Check sheet for the modelled part. Datum: model origin and axes. Units: mm. A direction names the side the tool comes from. Give positions to 0.01 mm unless a question says otherwise; leave off trailing zeros. Order: outer loops, then holes, each group sorted by start corner. A loop starts at its lowest first (then second) coordinate and runs counter-clockwise, first axis right, second up.
Autodesk Fusion 360 part; units mm, degrees
sketch "Esboço1" plane through (0, 0, 0) normal (0, 0, 1) x (1, 0, 0)
  circle A0 centre (0, 0) radius 3
  dimension "d1" = 6
extrude "Extrusão1" add sketch "Esboço1" along normal blind 40
sketch "Esboço2" plane through (0, 0, 40) normal (0, 0, 1) x (1, 0, 0)
  circle A0 centre (0, 0) radius 3
  circle A1 centre (0, 0) radius 2
  dimension "d4" = 4
extrude "Extrusão2" cut sketch "Esboço2" against normal blind 4 contours A1
extrude "Extrusão3" cut 1 faces at (-1.1591, 0.5829, 0) along direction (0, 0, 1) blind 10
extrude "Extrusão4" cut 1 faces at (0.637, 0.1965, 36) along direction (0, 0, -1) blind 1
chamfer "Chanfro1" distance 0.4 angle 45 1 edges at (-1.8647, 0.7232, 40)
sketch "Esboço3" plane through (0, 0, 10) normal (0, 0, -1) x (-1, 0, 0)
  circle A0 centre (0, 0) radius 3
  circle A1 centre (0, 0) radius 1.4
  dimension "d12" = 2.8
extrude "Extrusão5" cut sketch "Esboço3" against normal blind 10 contours A1
sketch "Esboço4" plane through (0, 0, 10) normal (0, 0, -1) x (-1, 0, 0)
  circle A0 centre (0, 0) radius 1.4
  circle A1 centre (0, 0) radius 3
  circle A2 centre (0, 0) radius 3
  circle A3 centre (0, 0) radius 2.75
  dimension "d15" = 5.5
extrude "Extrusão6" cut sketch "Esboço4" against normal blind 34 contours A1 A2
extrude "Extrusão7" cut 1 faces at (0.637, 0.1965, 35) along direction (0, 0, -1) blind 1
1) Material ranges on L1, parallel to Y at x = 0, z = 36.4; L2, parallel to Y at x = 0, z = 13.75; L3, parallel to Z at x = -1.5, y = 0.45, recorded low to high.
Recorded:
L1: y = -2.75 to -2, 2 to 2.75
L2: y = -2.75 to -1.4, 1.4 to 2.75
L3: z = 10 to 34
2) Section check C-C, the plane z = 33.25. Record the cut outline in (x, y).
Recorded:
outline: circle Ø5.5 at (0, 0)
3) Section check A-A, the plane x = 0. Record the cut outline in (y, z).
Recorded:
outline: (-2.75, 10) - (-1.4, 10) - (-1.4, 20) - (1.4, 20) - (1.4, 10) - (2.75, 10) - (2.75, 40) - (2.4, 40) - (2, 39.6) - (2, 34) - (-2, 34) - (-2, 39.6) - (-2.4, 40) - (-2.75, 40) - close
4) Section check D-D, the plane z = 12.5. Record the cut outline in (x, y), then the cut area to 3 significant figures.
Recorded:
outline: circle Ø5.5 at (0, 0); hole circle Ø2.8 at (0, 0)
area: 17.6 mm2
5) Draft check along X on faces 3 (the face through (0, 0, 20)), 4 (the face through (0.596, -2.685, 24.79)), 5 (the face through (1.2, -1.2, 10)). Enter one of: +X half, -X half, draft (parallel to the pull), parting line (faces both ways), or undercut.
Recorded:
face 3: undercut
face 4: parting line
face 5: draft
6) Set-up check for faces 1 (the face through (0, 0, 34)), 2 (the face through (1.4, 0.06, 14.93)): record each of +Z, -Z, +X, -X, +Y, -Y from which the full face is reachable in a straight line by a thin tool's end or side.
Recorded:
face 1: +Z
face 2: -Z
7) Depth check by flat-ended pin: pin 1 Ø1 at (x, z) = (-1, 24.5) entering from +Y; pin 2 Ø3 at (x, y) = (-0.5, 0.5) entering from +Z; pin 3 Ø1.7 at (x, y) = (0, 0) entering from +Z. Enter the tip coordinate at first touch or a pass-through.
Recorded:
pin 1: stops at y = 2.7
pin 2: stops at z = 39.81
pin 3: stops at z = 34
